from build123d import *

# Parameters (mm, degrees)
SKETCH1_R           = 13
SKETCH1_R_2         = 12
BOSS_EXTRUDE1_DEPTH = 10
SKETCH2_R           = 12
BOSS_EXTRUDE2_DEPTH = 170
SKETCH3_R           = 17
BOSS_EXTRUDE3_DEPTH = 2
SKETCH4_R           = 10
BOSS_EXTRUDE4_DEPTH = 12
CHAMFER1_SIZE       = 6
SKETCH5_W           = 10
SKETCH5_H           = 41
CUT_EXTRUDE1_DEPTH  = 20
CUT_EXTRUDE2_REACH  = 226.531


with BuildPart() as part:
    # Sketch1 → Boss-Extrude1 (new body)
    # profile 1 of 2: a face of its own
    with BuildSketch(Plane.XY):
        Circle(SKETCH1_R)
        Circle(SKETCH1_R_2, mode=Mode.SUBTRACT)
    # profile 2 of 2: a face of its own
    with BuildSketch(Plane.XY):
        Circle(SKETCH1_R_2)
    extrude(amount=BOSS_EXTRUDE1_DEPTH)

    # Sketch2 → Boss-Extrude2 (add)
    with BuildSketch(Plane.XY.offset(10)):
        Circle(SKETCH2_R)
    extrude(amount=BOSS_EXTRUDE2_DEPTH)

    # Sketch3 → Boss-Extrude3 (add)
    with BuildSketch(Plane.XY.offset(180)):
        Circle(SKETCH3_R)
    extrude(amount=BOSS_EXTRUDE3_DEPTH)

    # Sketch4 → Boss-Extrude4 (add, symmetric)
    with BuildSketch(Plane(origin=(0, 0, 0), x_dir=(0, 0, -1), z_dir=(1, 0, 0))):
        with BuildLine():
            Line((-182, 16), (-206, 16))
            ThreePointArc((-206, 16), (-222, 0), (-206, -16))
            Line((-206, -16), (-182, -16))
            Line((-182, -16), (-182, 16))
        make_face()
        with Locations((-206, 0)):
            Circle(SKETCH4_R, mode=Mode.SUBTRACT)
    extrude(amount=BOSS_EXTRUDE4_DEPTH, both=True)

    # Chamfer1
    # the kernel refuses this chamfer: 6 mm, written as the material it takes off along each edge
    with BuildSketch(Plane(origin=(12, 16, 182), x_dir=(0.027495876610586487, -0.9996219169112968, 0), z_dir=(0, 0, 1)), Plane(origin=(12, -16, 206), x_dir=(0.027495876610586487, 0.9996219169112968, 0), z_dir=(0, 0, -1)), Plane(origin=(-12, -16, 206), x_dir=(0.9996219169112968, -0.027495876610586202, 0), z_dir=(0, 0, -1))) as chamfer1_piece_1:
        Polygon((CHAMFER1_SIZE * 0.999621916911, -CHAMFER1_SIZE * 0.0274958766106), (-CHAMFER1_SIZE * 0.0274958766106, -CHAMFER1_SIZE * 0.999621916911), (0, 0), align=None)
    extrude(amount=24, mode=Mode.SUBTRACT)
    with BuildSketch(Plane(origin=(12, 0, 206), x_dir=(0, 1, 0), z_dir=(0, 0, -1))) as chamfer1_piece_2:
        Polygon((16 - CHAMFER1_SIZE, 0), (16, -CHAMFER1_SIZE), (16, 0), align=None)
    revolve(axis=Axis((12, 0, 206), (1, 0, 0)), revolution_arc=180, mode=Mode.SUBTRACT)
    with BuildSketch(Plane(origin=(-12, 16, 182), x_dir=(-0.027495876610586487, -0.9996219169112968, 0), z_dir=(0, 0, 1))) as chamfer1_piece_3:
        Polygon((CHAMFER1_SIZE * 0.999621916911, CHAMFER1_SIZE * 0.0274958766106), (-CHAMFER1_SIZE * 0.0274958766106, CHAMFER1_SIZE * 0.999621916911), (0, 0), align=None)
    extrude(amount=24, mode=Mode.SUBTRACT)
    with BuildSketch(Plane(origin=(-12, 0, 206), x_dir=(0, 1, 0), z_dir=(0, 0, -1))) as chamfer1_piece_4:
        Polygon((16 - CHAMFER1_SIZE, 0), (16, CHAMFER1_SIZE), (16, 0), align=None)
    revolve(axis=Axis((-12, 0, 206), (1, 0, 0)), revolution_arc=180, mode=Mode.SUBTRACT)

    # Sketch5 → Cut-Extrude1 (cut, symmetric)
    with BuildSketch(Plane(origin=(0, 0, 0), x_dir=(1, 0, 0), z_dir=(0, 1, 0))):
        with Locations((0, -202.5)):
            Rectangle(SKETCH5_W, SKETCH5_H)
    extrude(amount=CUT_EXTRUDE1_DEPTH, both=True, mode=Mode.SUBTRACT)

    # Cut-Extrude2: up to this face of the body (flat: up to its plane)
    cut_extrude2_end = Plane(part.part.faces().sort_by_distance((-12, 0, 190.227277531))[0])
    # Sketch6 → Cut-Extrude2 (cut, up to the picked face)
    with BuildSketch(Plane(origin=(12, 0, 0), x_dir=(0, 0, -1), z_dir=(1, 0, 0)), mode=Mode.PRIVATE) as cut_extrude2_sk1:
        with BuildLine():
            Line((-218.605812772, 9.853602608), (-213.878632982, 6.15850163))
            ThreePointArc((-213.878632982, 6.15850163), (-215.998555894, 0.169941286), (-214.083368787, -5.887202141))
            Line((-214.083368787, -5.887202141), (-218.35837697, -10.162210324))
            ThreePointArc((-218.35837697, -10.162210324), (-221.998777585, -0.197777146), (-218.605812772, 9.853602608))
        make_face()
    cut_extrude2_tool1 = split(extrude(cut_extrude2_sk1.sketch, amount=-CUT_EXTRUDE2_REACH, mode=Mode.PRIVATE), bisect_by=cut_extrude2_end, keep=Keep.BOTH, mode=Mode.PRIVATE)
    add(cut_extrude2_tool1.solids().sort_by(Axis((12, -0.027254, 218.293854), (-1, 0, 0)))[0], mode=Mode.SUBTRACT)


solid = part.part
The listing builds one solid part. Answer for the finished solid, in the listing's coordinates (mm). A direction names the side the tool comes from. Coordinates: 2 decimals unless noted, no trailing zeros. Write each loop counter-clockwise with the first axis right and the second up, starting at its lowest first coordinate (ties: lowest second). Pieces come first, ordered by that corner, then holes. Notation, with made-up numbers: M 51,9.5 L 95,9.5 A27 cw 95,34.5 Z; hole C -29.5,-24.5 d2. An arc over 180 degrees is marked long. Write each question's results on one line, items separated by ' | '.
Item 1: For a pull along Z with two mould halves and no side action, classify faces 4 (the face through (8.451, -0.519, 196.013)), 5 (the face through (4, 12, 180)), 6 (the face through (-10.316, -7.91, 4.93)), 7 (the face through (5.507, 14.426, 212.921)) as released by +Z, released by -Z, zero draft, split by the parting line, or undercut.
Answer below:
face 4: undercut | face 5: undercut | face 6: zero draft | face 7: released by +Z
Item 2: The part is cut by section A-A on z = 189. Determine the outline of the cut face in (x, y), and give its area (3 significant figures).
Answer below:
outline: M -12,-10 L -6,-16 L -5,-16 L -5,16 L -6,16 L -12,10 Z; M 5,-16 L 6,-16 L 12,-10 L 12,10 L 6,16 L 5,16 Z | area: 376 mm2
Item 3: Consider probe 1 along Z at (x, y) = (-11.5, -12); probe 2 along Z at (x, y) = (-8.25, 0); probe 3 along X at (y, z) = (-14, 194.5). Determine where each line is inside the solid, lowest interval first. Write a range as [from, to].
Answer below:
probe 1: [180, 182] | probe 2: [0, 196] | probe 3: [-8, -5], [5, 8]
Item 4: The part is cut by section B-B on y = 0. Determine the outline of the cut face in (x, z).
Answer below:
outline: M -17,180 L -12,180 L -12,10 L -13,10 L -13,0 L 13,0 L 13,10 L 12,10 L 12,180 L 17,180 L 17,182 L 12,182 L 12,196 L 5,196 L 5,182 L -5,182 L -5,196 L -12,196 L -12,182 L -17,182 Z
Item 5: Given P1, Ø0.8, axis at x = 5.5, z = 194, coming from the +Y side; P2, Ø6, axis at y = -3, z = 99, coming from the -X side; P3, Ø1, axis at x = -1, z = 25.5, coming from the +Y side; P4, Ø9.5, axis at y = -1, z = 201, coming from the +X side, each flat-ended and moving along its own axis, determine where each tip first touches the part or whether it passes through.
Answer below:
P1: y = 16 | P2: x = -12 | P3: y = 11.99 | P4: through
Item 6: The part is cut by section D-D on x = 9.5. Determine the outline of the cut face in (y, z), and give its area (3 significant figures).
Answer below:
outline: M -14.1,180 L -7.33,180 L -7.33,10 L -8.87,10 L -8.87,0 L 8.87,0 L 8.87,10 L 7.33,10 L 7.33,180 L 14.1,180 L 14.1,182 L 12.5,182 L 12.5,206 A12.5 ccw 7.7,215.85 L 6.16,213.88 A10 cw long -5.89,214.08 L -7.67,215.87 A12.5 ccw -12.5,206 L -12.5,182 L -14.1,182 Z | area: 3,220 mm2
Item 7: The part is cut by section C-C on x = 0. Determine the outline of the cut face in (y, z).
Answer below:
outline: M -17,180 L -12,180 L -12,10 L -13,10 L -13,0 L 13,0 L 13,10 L 12,10 L 12,180 L 17,180 L 17,182 L -17,182 Z
Item 8: Which of the six approach directions +Z, -Z, +X, -X, +Y, -Y give full straight-line access (tool end or side, diameter ignored) to faces 1 (the face through (9, -13, 194)), 2 (the face through (-12, 0, 189)), 3 (the face through (-7.67, 7.62, 215.75))?
Answer below:
face 1: +Z, +X, -Y | face 2: +Z, -X, +Y, -Y | face 3: +Z, +X, -X
